from build123d import *

# Parameters (mm, degrees)
BOSS_EXTRUDE1_DEPTH = 57
SKETCH2_W           = 42
SKETCH2_H           = 24
CUT_EXTRUDE1_DEPTH  = 1
SKETCH3_R           = 1.5
CUT_EXTRUDE2_DEPTH  = 2.54
SKETCH4_W           = 8.5
SKETCH4_H           = 24
CUT_EXTRUDE3_DEPTH  = 10
SKETCH5_R           = 1.5
CUT_EXTRUDE4_DEPTH  = 10
SKETCH6_W           = 40
SKETCH6_H           = 1
BOSS_EXTRUDE2_DEPTH = 5
SKETCH7_R           = 4
SKETCH7_R_2         = 1.5
CUT_EXTRUDE5_DEPTH  = 1
FILLET1_R           = 2


with BuildPart() as part:
    # Sketch1 → Boss-Extrude1 (new body)
    with BuildSketch(Plane.XY):
        Polygon((-46.692941858, 15.875), (-46.692941858, -8.125), (-16.692941858, -8.125), (-16.692941858, 15.875), (-17.692941858, 15.875), (-17.692941858, -7.125), (-45.692941858, -7.125), (-45.692941858, 15.875), align=None)
    extrude(amount=BOSS_EXTRUDE1_DEPTH)

    # Sketch2 → Cut-Extrude1 (cut)
    with BuildSketch(Plane(origin=(-16.692941858, 0, 0), x_dir=(0, 0, -1), z_dir=(1, 0, 0))):
        with Locations((-28.5, 3.875)):
            Rectangle(SKETCH2_W, SKETCH2_H)
    extrude(amount=-CUT_EXTRUDE1_DEPTH, mode=Mode.SUBTRACT)

    # Sketch3 → Cut-Extrude2 (cut)
    with BuildSketch(Plane(origin=(-16.692941858, 0, 0), x_dir=(0, 0, -1), z_dir=(1, 0, 0))):
        with Locations((-52.63, 11.176)):
            Circle(SKETCH3_R)
        with Locations((-4.37, 11.176)):
            Circle(SKETCH3_R)
        with Locations((-4.37, 1.016)):
            Circle(SKETCH3_R)
        with Locations((-52.63, 1.016)):
            Circle(SKETCH3_R)
    extrude(amount=-CUT_EXTRUDE2_DEPTH, mode=Mode.SUBTRACT)

    # Sketch4 → Cut-Extrude3 (cut)
    with BuildSketch(Plane.ZY.offset(46.692941858)):
        with Locations((4.25, 3.875)):
            Rectangle(SKETCH4_W, SKETCH4_H)
        with Locations((52.75, 3.875)):
            Rectangle(SKETCH4_W, SKETCH4_H)
    extrude(amount=-CUT_EXTRUDE3_DEPTH, mode=Mode.SUBTRACT)

    # Sketch5 → Cut-Extrude4 (cut)
    with BuildSketch(Plane.ZY.offset(46.692941858)):
        with Locations((38.5, 6.375)):
            Circle(SKETCH5_R)
        with Locations((18.5, 6.375)):
            Circle(SKETCH5_R)
    extrude(amount=-CUT_EXTRUDE4_DEPTH, mode=Mode.SUBTRACT)

    # Sketch6 → Boss-Extrude2 (add)
    with BuildSketch(Plane(origin=(-17.692941858, 0, 0), x_dir=(0, 0, -1), z_dir=(1, 0, 0))):
        with Locations((-28.5, -7.625)):
            Rectangle(SKETCH6_W, SKETCH6_H)
    extrude(amount=BOSS_EXTRUDE2_DEPTH)

    # Sketch7 → Cut-Extrude5 (cut)
    with BuildSketch(Plane(origin=(0, -8.125, 0), x_dir=(-1, 0, 0), z_dir=(0, -1, 0))):
        with Locations((24.692941858, -20)):
            Circle(SKETCH7_R)
        with Locations((24.692941858, -12)):
            Circle(SKETCH7_R_2)
        with Locations((32.692941858, -20)):
            Circle(SKETCH7_R_2)
        with Locations((24.692941858, -28)):
            Circle(SKETCH7_R_2)
        with Locations((16.692941858, -20)):
            Circle(SKETCH7_R_2)
        with Locations((32.692941858, -36)):
            Circle(SKETCH7_R_2)
        with Locations((24.692941858, -44)):
            Circle(SKETCH7_R_2)
        with Locations((16.692941858, -36)):
            Circle(SKETCH7_R_2)
        with Locations((24.692941858, -36)):
            Circle(SKETCH7_R)
    extrude(amount=-CUT_EXTRUDE5_DEPTH, mode=Mode.SUBTRACT)

    # Fillet1
    fillet1_edges = [part.edges().sort_by_distance(p)[0] for p in [
        (-12.692941858, -7.625, 8.5),
        (-12.692941858, -7.625, 48.5),
        (-17.192941858, 15.875, 57),
        (-36.692941858, -7.625, 0),
        (-46.192941858, 15.875, 8.5),
        (-45.692941858, -7.125, 28.5),
        (-46.692941858, -8.125, 28.5),
        (-36.692941858, -7.625, 57),
        (-17.192941858, 15.875, 0),
        (-46.192941858, 15.875, 48.5),
    ]]
    fillet(fillet1_edges, radius=FILLET1_R)


solid = part.part
Design review of the part built by this model. Coordinates are the model's own, in mm. A direction names the side the tool comes from. Coordinates: 2 decimals unless noted, no trailing zeros. Loops run counter-clockwise (first coordinate to the right, second up) from the corner with the lowest first, then second, coordinate; pieces in that order, holes last.
Item 1: Add section D-D (z = 36). Write out the cut boundary in (x, y) (3 decimals), and give its area (3 significant figures).
Completed:
outline: (-46.693, -6.125) arc R2 ccw to (-44.693, -8.125) - (-34.193, -8.125) - (-34.193, -7.125) - (-43.693, -7.125) arc R2 cw to (-45.693, -5.125) - (-45.693, 15.875) - (-46.693, 15.875) - close; (-31.193, -8.125) - (-28.693, -8.125) - (-28.693, -7.125) - (-31.193, -7.125) - close; (-20.693, -8.125) - (-18.193, -8.125) - (-18.193, -7.125) - (-20.693, -7.125) - close; (-15.193, -8.125) - (-12.693, -8.125) - (-12.693, -7.125) - (-15.193, -7.125) - close
area: 43.0 mm2
Item 2: Add section A-A (z = 4.37). Write out the cut boundary in (x, y) (3 decimals), and give its area (3 significant figures).
Completed:
outline: (-36.693, -8.125) - (-16.693, -8.125) - (-16.693, -0.484) - (-17.693, -0.484) - (-17.693, -7.125) - (-36.693, -7.125) - close; (-17.693, 2.516) - (-16.693, 2.516) - (-16.693, 9.676) - (-17.693, 9.676) - close; (-17.693, 12.676) - (-16.693, 12.676) - (-16.693, 15.875) - (-17.693, 15.875) - close
area: 37.0 mm2
Item 3: For faces 1 (the cylindrical face through (-32.368, -7.632, 37.464)), 2 (the flat face through (-46, 0, 48.5)), 3 (the flat face through (-46, 0, 8.5)), 4 (the cylindrical face through (-46.123, -7.524, 28.78)), 5 (the flat face through (-17.693, 5, 53)), list the 3-axis set-ups (+Z, -Z, +X, -X, +Y, -Y) from which the entire face can be reached by the end or side of a thin tool; tool diameter is ignored.
Completed:
face 1: +Y, -Y
face 2: +Z, -X, +Y, -Y
face 3: -Z, -X, +Y, -Y
face 4: +Z, -Z, -X, -Y
face 5: +Z, -Z, -X, +Y
Item 4: Wall thickness on L1, parallel to Y at x = -17.1, z = 52.63 (3 decimals); L2, parallel to Y at x = -33.5, z = 24 (3 decimals); L3, parallel to X at y = -7.5, z = 36: over which ranges is each line inside the solid? List them lowest first.
Completed:
L1: y = -8.125 to -0.484, 2.516 to 9.676, 12.676 to 15.875
L2: y = -8.125 to -7.125
L3: x = -46.15 to -34.19, -31.19 to -28.69, -20.69 to -18.19, -15.19 to -12.69
Item 5: Draft analysis for pull direction X (two halves, no side actions). For faces 6 (the flat face through (-17.693, 5, 4)), 7 (the cylindrical face through (-15.5, -7.63, 36.91)), 8 (the flat face through (-16.693, 4, 53)), state which applies: pulls with the +X half, pulls with the -X half, needs draft (parallel to the pull), parting line crosses it, or undercut.
Completed:
face 6: pulls with the -X half
face 7: undercut
face 8: pulls with the +X half
Item 6: Clearance check with flat-ended pins moving along their axes: pin 1 (2.5 mm diameter, centred on y = 1.016, z = 52.63, fed in from +X); pin 2 (8 mm diameter, centred on x = -36, y = -4.5, fed in from +Z); pin 3 (4 mm diameter, centred on x = -40.5, z = 33, fed in from +Y) (3 decimals); pin 4 (8 mm diameter, centred on y = 4, z = 53, fed in from -X). State where each tip first meets the part, or that it passes through.
Completed:
pin 1: passes through
pin 2: stops at z = 57
pin 3: stops at y = -7.125
pin 4: stops at x = -17.69
Item 7: Add section B-B (y = 9). Write out the cut boundary in (x, z), and give its area (3 significant figures).
Completed:
outline: (-46.69, 8.5) - (-45.69, 8.5) - (-45.69, 48.5) - (-46.69, 48.5) - close; (-17.69, 0) - (-16.69, 0) - (-16.69, 7.5) - (-17.69, 7.5) - close; (-17.69, 49.5) - (-16.69, 49.5) - (-16.69, 57) - (-17.69, 57) - close
area: 55.0 mm2
Item 8: Add section C-C (x = -22). Write out the cut boundary in (y, z) (3 decimals), and give its area (3 significant figures).
Completed:
outline: (-8.125, 0) - (-7.125, 0) - (-7.125, 17.042) - (-8.125, 17.042) - close; (-8.125, 22.958) - (-7.125, 22.958) - (-7.125, 33.042) - (-8.125, 33.042) - close; (-8.125, 38.958) - (-7.125, 38.958) - (-7.125, 57) - (-8.125, 57) - close
area: 45.2 mm2
